Study the drawing (mm; zero at the part's minimum x, y, z) and answer. A direction names the side the tool comes from. Give positions to 0.01 mm unless a question says otherwise; leave off trailing zeros. Order: outer loops, then holes, each group sorted by start corner. A loop starts at its lowest first (then second) coordinate and runs counter-clockwise, first axis right, second up.
Item 1: A cutting plane is placed at C-C (z = 12.5). Write down the section's boundary in (x, y), plus the area to 3 significant figures.
Item 2: A cutting plane is placed at A-A (x = 10.5). Write down the section's boundary in (y, z).
Item 3: Given pin 1 Ø8 at (x, y) = (17, 6.5) entering from -Z; pin 2 Ø12 at (y, z) = (11.5, 28.5) entering from +X; pin 3 Ø3 at (x, z) = (6.5, 12) entering from +Y; pin 4 Ø2.5 at (x, z) = (15.5, 43) entering from +Y, each flat-ended and moving along its own axis, determine where each tip first touches the part or whether it passes through.
Item 4: A cutting plane is placed at D-D (y = 9.5). Write down the section's boundary in (x, z).
Item 5: Find the intervals of material crossed by line 1 along Z through (x, y) = (2.75, 4.25); line 2 along X through (y, z) = (5.5, 12) (3 decimals); line 3 along Z through (x, y) = (7.75, 3.75), in increasing order.
Item 6: A cutting plane is placed at B-B (y = 13.25). Write down the section's boundary in (x, z), plus the area to 3 significant figures.
Item 7: Which of the six approach directions +Z, -Z, +X, -X, +Y, -Y give full straight-line access (tool end or side, diameter ignored) to the marked faces 1 and 2?
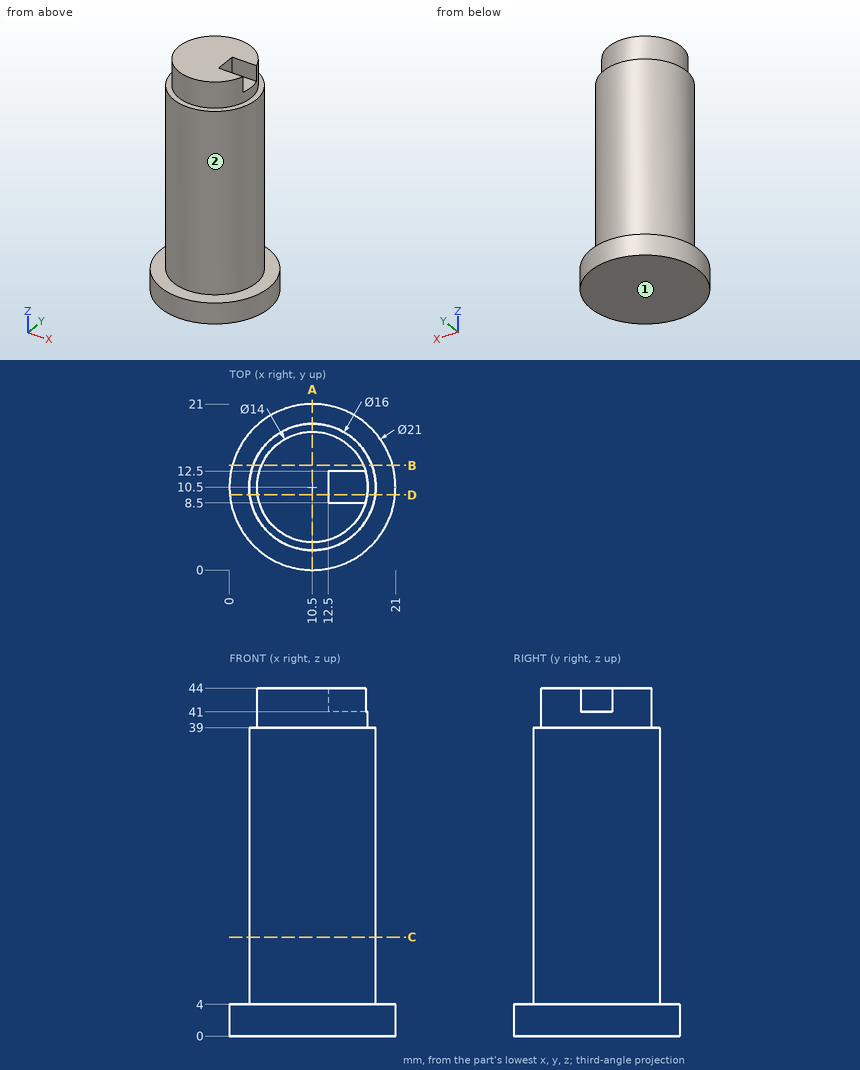
Response values:
1. outline: circle Ø16 at (10.5, 10.5)
1. area: 201 mm2
2. outline: (0, 0) - (21, 0) - (21, 4) - (18.5, 4) - (18.5, 39) - (17.5, 39) - (17.5, 44) - (3.5, 44) - (3.5, 39) - (2.5, 39) - (2.5, 4) - (0, 4) - close
3. pin 1: stops at z = 0
3. pin 2: stops at x = 18.5
3. pin 3: stops at y = 18.1
3. pin 4: stops at y = 16.41
4. outline: (0.05, 0) - (20.95, 0) - (20.95, 4) - (18.44, 4) - (18.44, 39) - (17.43, 39) - (17.43, 41) - (12.5, 41) - (12.5, 44) - (3.57, 44) - (3.57, 39) - (2.56, 39) - (2.56, 4) - (0.05, 4) - close
5. line 1: z = 0 to 4
5. line 2: x = 4.255 to 16.745
5. line 3: z = 0 to 39
6. outline: (0.37, 0) - (20.63, 0) - (20.63, 4) - (18.01, 4) - (18.01, 39) - (16.94, 39) - (16.94, 44) - (4.06, 44) - (4.06, 39) - (2.99, 39) - (2.99, 4) - (0.37, 4) - close
6. area: 671 mm2
7. face 1: -Z, +X, -X, +Y, -Y
7. face 2: +Z
